Read the model definition and answer for the solid it produces. Units are mm, in the model's axes. A direction names the side the tool comes from. Coordinates: 2 decimals unless noted, no trailing zeros. Loops run counter-clockwise (first coordinate to the right, second up) from the corner with the lowest first, then second, coordinate; pieces in that order, holes last. Notation, with made-up numbers: M 4.5,60.25 L 25.5,60.25 A19 ccw 25.5,80.25 Z; hole C 18,31 d9. An arc over 180 degrees is marked long. Use one line per item in the form item = value. Start each with the question number.
1. The part is cut by section A-A (x = 105). Give the vertices of the cut face in (y, z).
2. The part is cut by section B-B (z = 15.25). Give the vertices of the cut face in (x, y), plus the area to 3 significant figures.
3. The part is cut by section C-C (x = 15). Give the vertices of the cut face in (y, z).
4. The part is cut by section D-D (y = 2). Give the vertices of the cut face in (x, z), plus the area to 3 significant figures.
5. Flat-ended cylindrical pins translate along their axes: pin 1 (3 mm diameter, centred on x = 105, z = 10, fed in from +Y); pin 2 (9 mm diameter, centred on x = 16, y = 12.5, fed in from -Z); pin 3 (4 mm diameter, centred on x = 53.5, z = 13, fed in from +Y); pin 4 (5.5 mm diameter, centred on x = 104.5, z = 10, fed in from +Y). Find the tip coordinate at first contact, or state that the pin passes through.
6. For a pull along Z with two mould halves and no side action, classify faces 5 (the cylindrical face through (27.85, 17.32, 19.1)), 6 (the flat face through (79, 4, 0)), 7 (the flat face through (0, 18, 10)), 8 (the cylindrical face through (7.921, 6.337, 10.845)) as released by +Z, released by -Z, zero draft, split by the parting line, or undercut.
7. Find the intervals of material crossed by probe 1 along Z at (x, y) = (7, 9.5); probe 2 along Y at (x, z) = (102.5, 16.5); probe 3 along X at (y, z) = (21.5, 10.75), in increasing order. Write a range as [from, to].
8. A tool of negligible diameter and unlimited length cuts with its end or side. For faces 1 (the cylindrical face through (103.331, 17.303, 10.526)), 2 (the flat face through (108, 13.5, 10)), 3 (the flat face through (56, 6.977, 10)), 4 (the cylindrical face through (84.1, 17.2, 0.9)), from which of +Z, -Z, +X, -X, +Y, -Y can it reach the whole face along a straight path? Write none if from no direction.
from build123d import *

# Parameters (mm, degrees)
F1_DEPTH  = 20
F2_R      = 3
F3_R      = 1.25
F4_DEPTH  = 30
F3_R_2    = 1.75
F5_DEPTH  = 12
F3_R_3    = 3.5
F6_DEPTH  = 4
F7_R      = 1.25
F8_DEPTH  = 30
F7_R_2    = 1.75
F9_DEPTH  = 12
F7_R_3    = 3.5
F10_DEPTH = 4


# Not quite as in the source:
# - a feature names something its author has since deleted; it is built from what else it names


with BuildPart() as f1:
    # F0 (on Top) → F1 (new body)
    with BuildSketch(Plane.XY):
        with BuildLine():
            Line((3, 0), (56, 0))
            Line((56, 0), (109, 0))
            ThreePointArc((109, 0), (111.1213203436, 0.8786796564), (112, 3))
            Line((112, 3), (112, 12.5))
            Line((112, 12.5), (101, 12.5))
            ThreePointArc((101, 12.5), (91.025319235, 11.99745519), (100.8989794856, 13.5))
            Line((100.8989794856, 13.5), (112, 13.5))
            Line((112, 13.5), (112, 22))
            ThreePointArc((112, 22), (111.1213203436, 24.1213203436), (109, 25))
            Line((109, 25), (95.7940161003, 25))
            Line((95.7940161003, 25), (92, 25))
            Line((92, 25), (89.649228215, 25))
            ThreePointArc((89.649228215, 25), (86.8322254301, 24.1309194267), (84.9945036033, 21.825798124))
            Line((84.9945036033, 21.825798124), (81.660193975, 13.3252454689))
            ThreePointArc((81.660193975, 13.3252454689), (77.9847503214, 8.7150028635), (72.3507447516, 6.9768417168))
            Line((72.3507447516, 6.9768417168), (61.9619729666, 6.9768417168))
            Line((61.9619729666, 6.9768417168), (56, 6.9768417168))
            Line((56, 6.9768417168), (50.0380270334, 6.9768417168))
            Line((50.0380270334, 6.9768417168), (39.6492552484, 6.9768417168))
            ThreePointArc((39.6492552484, 6.9768417168), (34.0152496786, 8.7150028635), (30.339806025, 13.3252454689))
            Line((30.339806025, 13.3252454689), (27.0054963967, 21.825798124))
            ThreePointArc((27.0054963967, 21.825798124), (25.1677745699, 24.1309194267), (22.350771785, 25))
            Line((22.350771785, 25), (20, 25))
            Line((20, 25), (16.2059838997, 25))
            Line((16.2059838997, 25), (3, 25))
            ThreePointArc((3, 25), (0.8786796564, 24.1213203436), (0, 22))
            Line((0, 22), (0, 13.5))
            Line((0, 13.5), (11.1010205144, 13.5))
            ThreePointArc((11.1010205144, 13.5), (20.974680765, 11.99745519), (11, 12.5))
            Line((11, 12.5), (0, 12.5))
            Line((0, 12.5), (0, 3))
            ThreePointArc((0, 3), (0.8786796564, 0.8786796564), (3, 0))
        make_face()
    extrude(amount=F1_DEPTH)

    # F2
    f2_edges = [f1.edges().sort_by_distance(p)[0] for p in [
        (56, 0, 20),
        (99.324614, 25, 20),
        (56, 0, 0),
        (99.324614, 25, 0),
    ]]
    fillet(f2_edges, radius=F2_R)

    # F3 (on face) → F4 (cut)
    with BuildSketch(Plane(origin=(0, 25, 0), x_dir=(-1, 0, 0), z_dir=(0, 1, 0))):
        with Locations((-7, 10)):
            Circle(F3_R)
    extrude(amount=-F4_DEPTH, mode=Mode.SUBTRACT)

    # F3 (on face) → F5 (cut)
    with BuildSketch(Plane(origin=(0, 25, 0), x_dir=(-1, 0, 0), z_dir=(0, 1, 0))):
        with Locations((-7, 10)):
            Circle(F3_R_2)
        with Locations((-7, 10)):
            Circle(F3_R, mode=Mode.SUBTRACT)
    extrude(amount=-F5_DEPTH, mode=Mode.SUBTRACT)

    # F3 (on face) → F6 (cut)
    with BuildSketch(Plane(origin=(0, 25, 0), x_dir=(-1, 0, 0), z_dir=(0, 1, 0))):
        with Locations((-7, 10)):
            Circle(F3_R_3)
        with Locations((-7, 10)):
            Circle(F3_R_2, mode=Mode.SUBTRACT)
        with Locations((-7, 10)):
            Circle(F3_R_2)
        with Locations((-7, 10)):
            Circle(F3_R, mode=Mode.SUBTRACT)
        with Locations((-7, 10)):
            Circle(F3_R)
    extrude(amount=-F6_DEPTH, mode=Mode.SUBTRACT)

    # F7 (on face) → F8 (cut)
    with BuildSketch(Plane(origin=(0, 25, 0), x_dir=(-1, 0, 0), z_dir=(0, 1, 0))):
        with Locations((-105, 10)):
            Circle(F7_R)
    extrude(amount=-F8_DEPTH, mode=Mode.SUBTRACT)

    # F7 (on face) → F9 (cut)
    with BuildSketch(Plane(origin=(0, 25, 0), x_dir=(-1, 0, 0), z_dir=(0, 1, 0))):
        with Locations((-105, 10)):
            Circle(F7_R_2)
        with Locations((-105, 10)):
            Circle(F7_R, mode=Mode.SUBTRACT)
    extrude(amount=-F9_DEPTH, mode=Mode.SUBTRACT)

    # F7 (on face) → F10 (cut)
    with BuildSketch(Plane(origin=(0, 25, 0), x_dir=(-1, 0, 0), z_dir=(0, 1, 0))):
        with Locations((-105, 10)):
            Circle(F7_R_3)
        with Locations((-105, 10)):
            Circle(F7_R_2, mode=Mode.SUBTRACT)
    extrude(amount=-F10_DEPTH, mode=Mode.SUBTRACT)


solid = f1.part
Computed values:
q1.outline = M 0,3 A3 ccw 3,0 L 12.5,0 L 12.5,8.75 L 0,8.75 Z; M 0,11.25 L 12.5,11.25 L 12.5,20 L 3,20 A3 ccw 0,17 Z; M 13.5,0 L 22,0 A3 ccw 25,3 L 25,6.5 L 21,6.5 L 21,8.25 L 13.5,8.25 Z; M 13.5,11.75 L 21,11.75 L 21,13.5 L 25,13.5 L 25,17 A3 ccw 22,20 L 13.5,20 Z
q2.outline = M 0,3 A3 ccw 3,0 L 109,0 A3 ccw 112,3 L 112,12.5 L 101,12.5 A5 cw long 100.9,13.5 L 112,13.5 L 112,22 A3 ccw 109,25 L 89.65,25 A5 ccw 84.99,21.83 L 81.66,13.33 A10 cw 72.35,6.98 L 39.65,6.98 A10 cw 30.34,13.33 L 27.01,21.83 A5 ccw 22.35,25 L 3,25 A3 ccw 0,22 L 0,13.5 L 11.1,13.5 A5 cw long 11,12.5 L 0,12.5 Z
q2.area = 1,660 mm²
q3.outline = M 0,3 A3 ccw 3,0 L 7.6,0 L 7.6,20 L 3,20 A3 ccw 0,17 Z; M 17.4,0 L 22,0 A3 ccw 25,3 L 25,17 A3 ccw 22,20 L 17.4,20 Z
q4.outline = M 0.17,3 A2.83 ccw 3,0.17 L 109,0.17 A2.83 ccw 111.83,3 L 111.83,17 A2.83 ccw 109,19.83 L 3,19.83 A2.83 ccw 0.17,17 Z; hole C 7,10 d2.5; hole C 105,10 d2.5
q4.area = 2,180 mm²
q5.pin_1 = 12.5
q5.pin_2 = through
q5.pin_3 = 6.98
q5.pin_4 = 21
q6.face_5 = released by +Z
q6.face_6 = released by -Z
q6.face_7 = zero draft
q6.face_8 = undercut
q7.probe_1 = [0, 8.75], [11.25, 20]
q7.probe_2 = [0, 12.5], [13.5, 25]
q7.probe_3 = [0, 3.58], [10.42, 27.13], [84.87, 101.58], [108.42, 112]
q8.face_1 = +Y
q8.face_2 = +Z, -Z, +X
q8.face_3 = +Z, -Z, +Y
q8.face_4 = -Z, +Y
